```python
from build123d import *

# Parameters (mm, degrees)
ESQUISSE1_W             = 40
ESQUISSE1_H             = 8
BOSS_EXTRU_1_DEPTH      = 8
ESQUISSE2_W             = 20
ESQUISSE2_H             = 8
BOSS_EXTRU_2_DEPTH      = 12
CONG_1_R                = 2
ESQUISSE3_R             = 2.1
ENL_V_MAT_EXTRU_1_DEPTH = 9
ESQUISSE5_R             = 1.6
ENL_V_MAT_EXTRU_2_DEPTH = 21
ESQUISSE6_R             = 7
ENL_V_MAT_EXTRU_3_DEPTH = 3


with BuildPart() as part:
    # Esquisse1 → Boss.-Extru.1 (new body)
    with BuildSketch(Plane.XY):
        with Locations((20, 4)):
            Rectangle(ESQUISSE1_W, ESQUISSE1_H)
    extrude(amount=BOSS_EXTRU_1_DEPTH)

    # Esquisse2 → Boss.-Extru.2 (add)
    with BuildSketch(Plane.XY.offset(8)):
        with Locations((10, 4)):
            Rectangle(ESQUISSE2_W, ESQUISSE2_H)
    extrude(amount=BOSS_EXTRU_2_DEPTH)

    # Congé1
    cong_1_edges = [part.edges().sort_by_distance(p)[0] for p in [
        (0, 4, 0),
        (40, 4, 8),
        (0, 4, 20),
        (20, 4, 20),
        (20, 4, 8),
    ]]
    fillet(cong_1_edges, radius=CONG_1_R)

    # Esquisse3 → Enlèv. mat.-Extru.1 (cut, through all)
    with BuildSketch(Plane(origin=(0, 8, 0), x_dir=(1, 0, 0), z_dir=(0, 1, 0))):
        with Locations((10, -10)):
            Circle(ESQUISSE3_R)
    extrude(amount=-ENL_V_MAT_EXTRU_1_DEPTH, mode=Mode.SUBTRACT)

    # Esquisse5 → Enlèv. mat.-Extru.2 (cut, through all)
    with BuildSketch(Plane(origin=(0, 0, 0), x_dir=(-1, 0, 0), z_dir=(0, 0, -1))):
        with Locations((-30.6, 4)):
            Circle(ESQUISSE5_R)
    extrude(amount=-ENL_V_MAT_EXTRU_2_DEPTH, mode=Mode.SUBTRACT)

    # Esquisse6 → Enlèv. mat.-Extru.3 (cut)
    with BuildSketch(Plane(origin=(0, 8, 0), x_dir=(1, 0, 0), z_dir=(0, 1, 0))):
        with Locations((10, -10)):
            Circle(ESQUISSE6_R)
    extrude(amount=-ENL_V_MAT_EXTRU_3_DEPTH, mode=Mode.SUBTRACT)


solid = part.part
```
Verification items for the finished model (mm, model axes). A direction names the side the tool comes from. Round coordinates to 2 decimals unless told otherwise and drop trailing zeros. Order: outer loops, then holes, each group sorted by start corner. A loop starts at its lowest first (then second) coordinate and runs counter-clockwise, first axis right, second up.
1) Material ranges on line 1 (Z direction, x = 10, y = 2.65); line 2 (X direction, y = 5.75, z = 10), recorded low to high.
Geometry says:
line 1: z = 0 to 7.9, 12.1 to 20
line 2: x = 0 to 3, 17 to 20
2) Cross-section at C-C, the plane y = 7.25. Record the cut outline in (x, z), plus the area to 3 significant figures.
Geometry says:
outline: (0, 2) arc R2 ccw to (2, 0) - (40, 0) - (40, 6) arc R2 ccw to (38, 8) - (22, 8) arc R2 cw to (20, 10) - (20, 18) arc R2 ccw to (18, 20) - (2, 20) arc R2 ccw to (0, 18) - close; hole circle Ø14 at (10, 10)
area: 403 mm2
3) Cross-section at D-D, the plane z = 4. Record the cut outline in (x, y).
Geometry says:
outline: (0, 0) - (40, 0) - (40, 8) - (13.61, 8) - (13.61, 5) - (6.39, 5) - (6.39, 8) - (0, 8) - close; hole circle Ø3.2 at (30.6, 4)
4) Cross-section at A-A, the plane x = 10. Record the cut outline in (y, z).
Geometry says:
outline: (0, 0) - (8, 0) - (8, 3) - (5, 3) - (5, 7.9) - (0, 7.9) - close; (0, 12.1) - (5, 12.1) - (5, 17) - (8, 17) - (8, 20) - (0, 20) - close
5) Draft check along X on faces 1 (the cylindrical face through (29, 4, 4)), 2 (the flat face through (28, 4, 8)), 3 (the flat face through (40, 4, 3)), 4 (the flat face through (8.3, 5, 11.5)). Enter one of: +X half, -X half, draft (parallel to the pull), parting line (faces both ways), or undercut.
Geometry says:
face 1: undercut
face 2: draft
face 3: +X half
face 4: undercut
6) Cross-section at B-B, the plane y = 3. Record the cut outline in (x, z), plus the area to 3 significant figures.
Geometry says:
outline: (0, 2) arc R2 ccw to (2, 0) - (29.35, 0) - (29.35, 8) - (22, 8) arc R2 cw to (20, 10) - (20, 18) arc R2 ccw to (18, 20) - (2, 20) arc R2 ccw to (0, 18) - close; (31.85, 0) - (40, 0) - (40, 6) arc R2 ccw to (38, 8) - (31.85, 8) - close; hole circle Ø4.2 at (10, 10)
area: 524 mm2
7) Tool access check on faces 5 (the flat face through (10, 4, 20)), 6 (the flat face through (20, 4, 14)), 7 (the cylindrical face through (16.466, 6.521, 12.681)). Record the directions out of +Z, -Z, +X, -X, +Y, -Y that give a thin tool (end or side, any length) a straight path to the whole face; none if there is none.
Geometry says:
face 5: +Z, +X, -X, +Y, -Y
face 6: +Z, +X, +Y, -Y
face 7: +Y
